```python
from build123d import *

# Parameters (mm, degrees)
F0_W     = 5
F0_H     = 5
F0_W_2   = 10
F1_DEPTH = 20
F2_DEPTH = 10
F3_R     = 5
F5_DEPTH = 5
F7_DEPTH = 50
F9_DEPTH = 5


with BuildPart() as f1:
    # F0 (on Top) → F1 (new body)
    with BuildSketch(Plane.XY):
        Polygon((-46.9086258113, 17.5), (-46.9086258113, 0), (98.0913741887, 0), (98.0913741887, 45), (-46.9086258113, 45), (-46.9086258113, 27.5), align=None)
        with Locations((-24.4086258113, 22.5)):
            Rectangle(F0_W, F0_H, mode=Mode.SUBTRACT)
        with Locations((3.0913741887, 22.5)):
            Rectangle(F0_W_2, F0_H, mode=Mode.SUBTRACT)
        Polygon((28.0913741887, 10), (28.0913741887, 25), (28.0913741887, 35), (33.0913741887, 35), (33.0913741887, 10), align=None, mode=Mode.SUBTRACT)
    extrude(amount=F1_DEPTH)

    # F0 (on Top) → F2 (join)
    with BuildSketch(Plane.XY):
        with Locations((-24.4086258113, 22.5)):
            Rectangle(F0_W, F0_H)
        with Locations((3.0913741887, 22.5)):
            Rectangle(F0_W_2, F0_H)
    extrude(amount=F2_DEPTH)

    # F3
    f3_edges = [f1.edges().sort_by_distance(p)[0] for p in [
        (33.091374, 22.5, 20),
        (28.091374, 22.5, 20),
        (28.091374, 22.5, 0),
        (33.091374, 22.5, 0),
    ]]
    fillet(f3_edges, radius=F3_R)

    # F4 (on face) → F5 (join)
    with BuildSketch(Plane.XY.offset(20)):
        Polygon((-46.9086258113, 17.5), (-46.9086258113, 27.5), (-49.4086258113, 27.5), (-49.4086258113, 30), (-54.4086258113, 30), (-54.4086258113, 15), (-49.4086258113, 15), (-49.4086258113, 17.5), align=None)
    extrude(amount=-F5_DEPTH)

    # F6 (on face) → F7 (cut)
    with BuildSketch(Plane.XZ):
        Polygon((93.9913741887, 10), (83.0913741887, 10), (83.0913741887, 15), (78.0913741887, 15), (78.0913741887, 0), (98.0913741887, 0), (98.0913741887, 5.01), (93.9913741887, 5.01), align=None)
    extrude(amount=-F7_DEPTH, mode=Mode.SUBTRACT)

    # F8 (on face) → F9 (cut)
    with BuildSketch(Plane.XY.offset(20)):
        Polygon((48.0913741887, 0), (68.0913741887, 0), (68.0913741887, 5), (73.0913741887, 5), (73.0913741887, 15), (43.0913741887, 15), (43.0913741887, 5), (48.0913741887, 5), align=None)
        Polygon((68.0913741887, 40), (68.0913741887, 45), (48.0913741887, 45), (48.0913741887, 40), (43.0913741887, 40), (43.0913741887, 30), (73.0913741887, 30), (73.0913741887, 40), align=None)
    extrude(amount=-F9_DEPTH, mode=Mode.SUBTRACT)


solid = f1.part
```
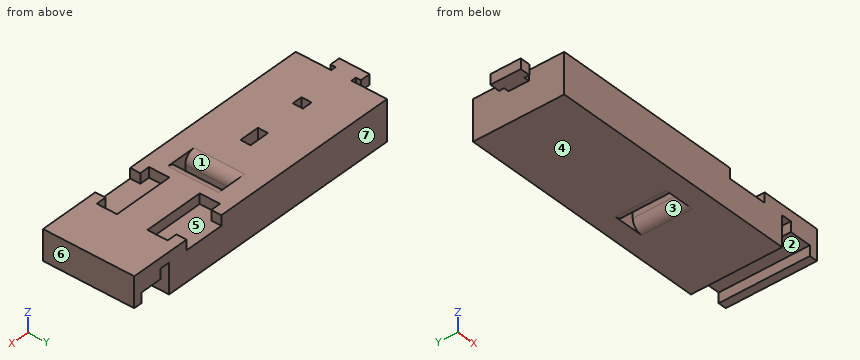
Build history of the part. All positions in model axes, mm. Face numbers are marked on the shaded views. A direction names the side the tool comes from. Coordinates: 2 decimals unless noted, no trailing zeros. Order: outer loops, then holes, each group sorted by start corner. A loop starts at its lowest first (then second) coordinate and runs counter-clockwise, first axis right, second up. Notation, with made-up numbers: (76.25, 86) -> (106.25, 86) arc R21 cw to (106.25, 108) -> close; hole circle Ø10 at (85.25, 23.25). An arc over 180 degrees is marked (long way). Answer in a Markdown table with one row per item. Add a question column.
Q1. Band-saw the part on B-B, the plane y = 38.5. List the corners of the cut face in (x, z), then the cut area to 3 significant figures.
Q2. Band-saw the part on C-C, the plane x = -24. List the corners of the cut face in (y, z), then the cut area to 3 significant figures.
Q3. Which spindle directions (+Z, -Z, +X, -X, +Y, -Y) get a long thin tool onto all of the face, cutting with end or side? Do the marked faces 1, 2, 3 and 4. Say none if no direction does.
Q4. Wall check: line 1 along X through (y, z) = (22.5, 10.75); line 2 along X through (y, z) = (13, 11.75); line 3 along X through (y, z) = (20.5, 7). Give the ranges that are in metal, low to high. Write a range as [from, to].
Q5. Drop flat-ended pins along their axis: pin 1 (1.5 mm diameter, centred on y = 36, z = 17, fed in from -X); pin 2 (4 mm diameter, centred on x = -51.5, y = 22, fed in from -Z). Give the stop position or say it passes through.
Q6. Band-saw the part on A-A, the plane z = 7.5. List the corners of the cut face in (x, y).
Q7. Band-saw the part on D-D, the plane z = 18.5. Give the number of separate pieces and of enclosed holes in the cut face, then the cut area to 3 significant figures.
Q8. Mould opens along X. For the marked faces 5, 6 and 7 say: +X half, -X half, draft (parallel to the pull), parting line (faces both ways), or undercut.
Answers follow:
| question | item | result |
|---|---|---|
| 1 | outline | (-46.91, 0) -> (78.09, 0) -> (78.09, 15) -> (83.09, 15) -> (83.09, 10) -> (93.99, 10) -> (93.99, 5.01) -> (98.09, 5.01) -> (98.09, 20) -> (73.09, 20) -> (73.09, 15) -> (43.09, 15) -> (43.09, 20) -> (-46.91, 20) -> close |
| 1 | area | 2,550 mm^2 |
| 2 | outline | (0, 0) -> (45, 0) -> (45, 20) -> (25, 20) -> (25, 10) -> (20, 10) -> (20, 20) -> (0, 20) -> close |
| 2 | area | 850 mm^2 |
| 3 | face 1 | +Z |
| 3 | face 2 | -Z, +Y, -Y |
| 3 | face 3 | -Z |
| 3 | face 4 | -Z, +X, -X, +Y, -Y |
| 4 | line 1 | [-46.91, -26.91], [-21.91, -1.91], [8.09, 28.09], [33.09, 78.09], [83.09, 98.09] |
| 4 | line 2 | [-46.91, 28.09], [33.09, 78.09], [83.09, 98.09] |
| 4 | line 3 | [-46.91, 28.09], [33.09, 78.09], [93.99, 98.09] |
| 5 | pin 1 | x = -46.91 |
| 5 | pin 2 | z = 15 |
| 6 | outline | (-46.91, 0) -> (78.09, 0) -> (78.09, 45) -> (-46.91, 45) -> close; (93.99, 0) -> (98.09, 0) -> (98.09, 45) -> (93.99, 45) -> close; hole (28.09, 10) -> (33.09, 10) -> (33.09, 35) -> (28.09, 35) -> close |
| 7 | separate pieces | 1 |
| 7 | enclosed holes | 3 |
| 7 | area | 5,550 mm^2 |
| 8 | face 5 | undercut |
| 8 | face 6 | +X half |
| 8 | face 7 | draft |
